Study the drawing (mm; zero at the part's minimum x, y, z) and answer. Coordinates: 2 decimals unless noted, no trailing zeros. Loops run counter-clockwise (first coordinate to the right, second up) from the corner with the lowest first, then second, coordinate; pieces in that order, holes last. Notation, with made-up numbers: (-20.5, 30.25) -> (-16.5, 30.25) arc R23 cw to (-16.5, 56.25) -> close; hole circle Ø1 at (48.25, 43.5). An arc over 180 degrees is marked (long way). Answer in a Markdown table with one row per item.
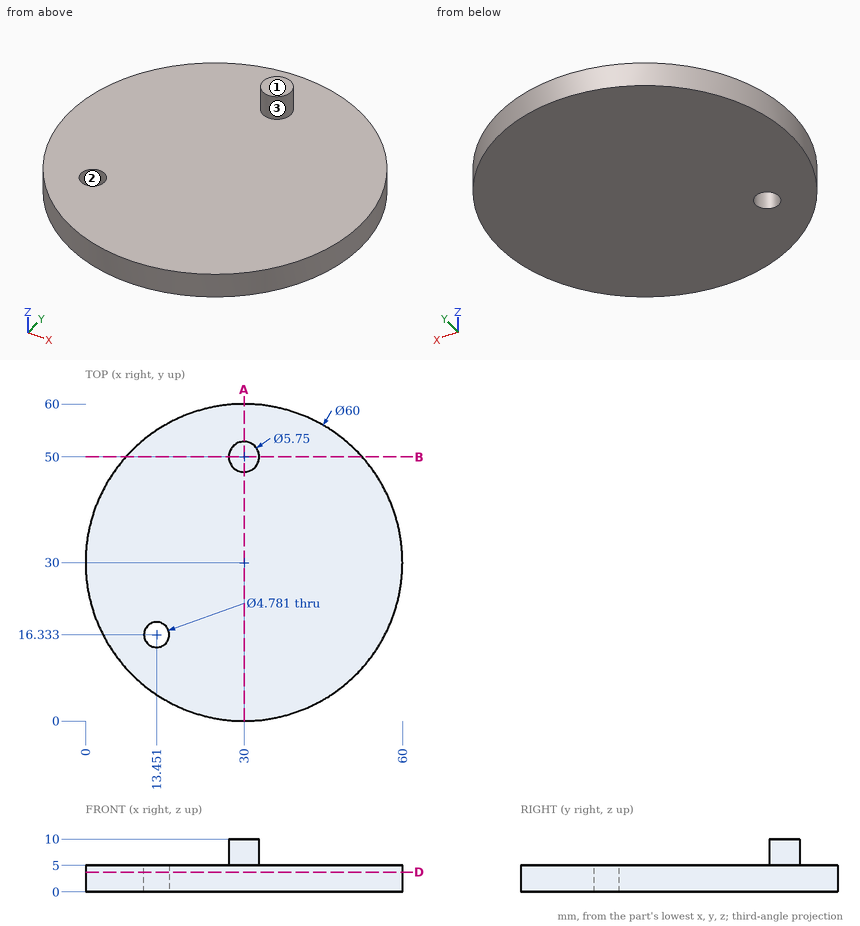
1. Find the intervals of material crossed by probe 1 along Z at (x, y) = (16, 13); probe 2 along Y at (x, z) = (52, 1) (1 decimal); probe 3 along Y at (x, z) = (47, 1.5), in increasing order.
A:
| item | result |
|---|---|
| probe 1 | z = 0 to 5 |
| probe 2 | y = 9.6 to 50.4 |
| probe 3 | y = 5.28 to 54.72 |
2. A cutting plane is placed at A-A on x = 30. Give the vertices of the cut face in (y, z) (1 decimal).
A:
| item | result |
|---|---|
| outline | (0, 0) -> (60, 0) -> (60, 5) -> (52.9, 5) -> (52.9, 10) -> (47.1, 10) -> (47.1, 5) -> (0, 5) -> close |
3. The mould has two halves that part along Y. Classify the marked faces 1, 2 and 3: pulls with the +Y half, pulls with the -Y half, needs draft (parallel to the pull), parting line crosses it, or undercut.
A:
| item | result |
|---|---|
| face 1 | needs draft |
| face 2 | undercut |
| face 3 | parting line crosses it |
4. Given pin 1 Ø6 at (x, y) = (13.45, 16.33) entering from +Z; pin 2 Ø5 at (y, z) = (48.5, 2.5) entering from -X, each flat-ended and moving along its own axis, determine where each tip first touches the part or whether it passes through.
A:
| item | result |
|---|---|
| pin 1 | stops at z = 5 |
| pin 2 | stops at x = 4.62 |
5. A cutting plane is placed at B-B on y = 50. Give the vertices of the cut face in (x, z) (1 decimal), and give its area (3 significant figures).
A:
| item | result |
|---|---|
| outline | (7.6, 0) -> (52.4, 0) -> (52.4, 5) -> (32.9, 5) -> (32.9, 10) -> (27.1, 10) -> (27.1, 5) -> (7.6, 5) -> close |
| area | 252 mm2 |
6. A cutting plane is placed at D-D on z = 3.75. Give the vertices of the cut face in (x, y).
A:
| item | result |
|---|---|
| outline | circle Ø60 at (30, 30); hole circle Ø4.78 at (13.45, 16.33) |
